Geometry check sheet. Reference: drawing and pictorial views, mm from the part's lowest x, y, z. A direction names the side the tool comes from. Coordinates: 2 decimals unless noted, no trailing zeros. Loops run counter-clockwise (first coordinate to the right, second up) from the corner with the lowest first, then second, coordinate; pieces in that order, holes last. Notation, with made-up numbers: (-23.5, 84) - (-9.5, 84) arc R28 cw to (-9.5, 104) - close; hole circle Ø3 at (26.5, 38.25). An arc over 180 degrees is marked (long way). Use a Markdown table: item, result. Add a question column.
1) Thickness scan on line 1 (X direction, y = 7.75, z = 2.75); line 2 (Y direction, x = 42.5, z = 11) (1 decimal); line 3 (Z direction, x = 93.5, y = 8.25) (1 decimal). Record the ranges inside material, lowest first.
2) Go/stop test with flat-tipped pins: P1, Ø6, axis at x = 77.5, y = 7.5, coming from the +Z side (1 decimal); P2, Ø4, axis at x = 34.5, y = 9, coming from the -Z side (1 decimal); P3, Ø4, axis at x = 15.5, y = 8.5, coming from the +Z side; P4, Ø3, axis at x = 80.5, y = 4, coming from the +Z side (1 decimal). Record where each tip stops, or that it passes through.
3) Sectioned sample at B-B, the plane z = 7. Enter the section's corners in (x, y), then the cut area to 3 significant figures.
4) Sectioned sample at D-D, the plane z = 1. Enter the section's corners in (x, y).
5) Tool access check on the marked faces 1, 2 and 3. Record the directions out of +Z, -Z, +X, -X, +Y, -Y that give a thin tool (end or side, any length) a straight path to the whole face; none if there is none.
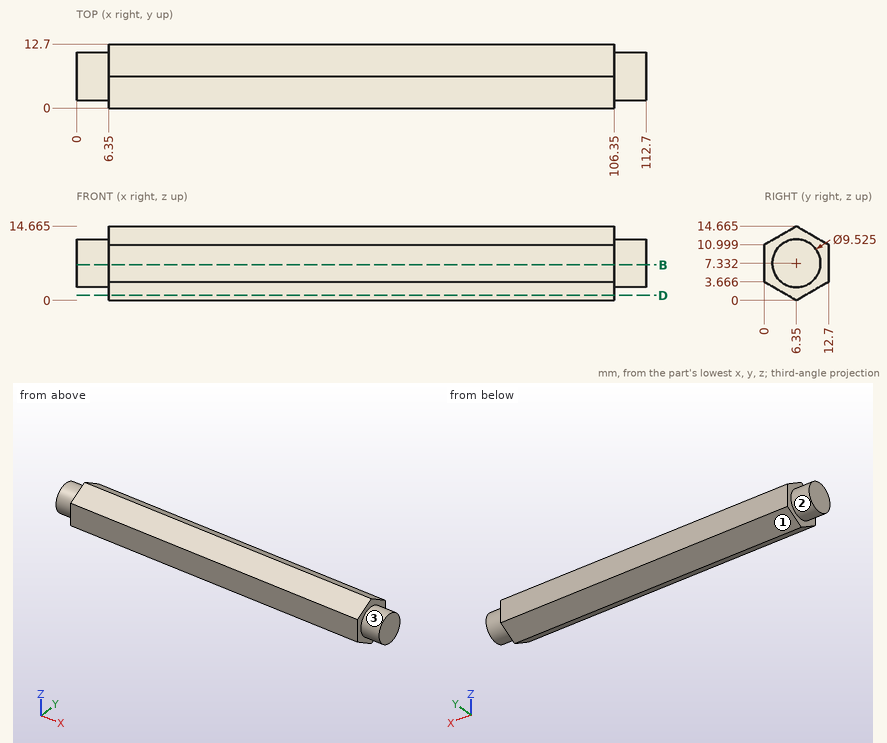
Solved:
| question | item | result |
|---|---|---|
| 1 | line 1 | x = 6.35 to 106.35 |
| 1 | line 2 | y = 0 to 12.7 |
| 1 | line 3 | z = 1.1 to 13.6 |
| 2 | P1 | stops at z = 14.7 |
| 2 | P2 | stops at z = 0.4 |
| 2 | P3 | stops at z = 14.58 |
| 2 | P4 | stops at z = 14.2 |
| 3 | outline | (0, 1.6) - (6.35, 1.6) - (6.35, 0) - (106.35, 0) - (106.35, 1.6) - (112.7, 1.6) - (112.7, 11.1) - (106.35, 11.1) - (106.35, 12.7) - (6.35, 12.7) - (6.35, 11.1) - (0, 11.1) - close |
| 3 | area | 1,390 mm2 |
| 4 | outline | (6.35, 4.62) - (106.35, 4.62) - (106.35, 8.08) - (6.35, 8.08) - close |
| 5 | face 1 | -Z, +X, -X, +Y |
| 5 | face 2 | -X |
| 5 | face 3 | +X |
